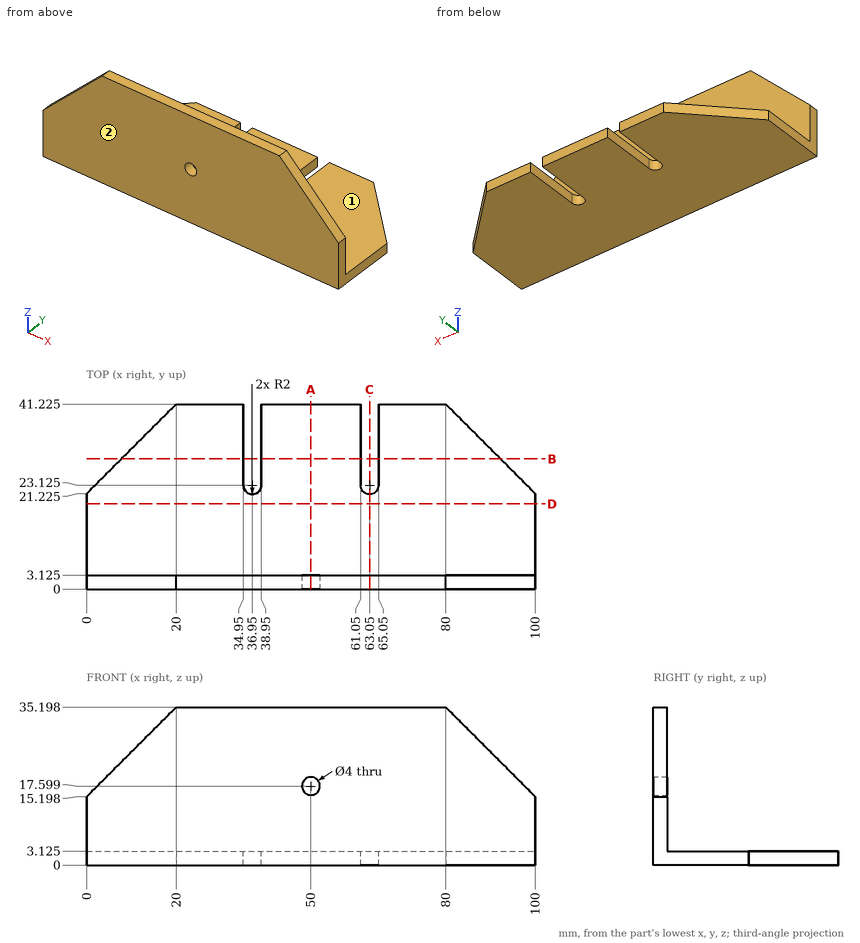
Geometry check sheet. Reference: drawing and pictorial views, mm from the part's lowest x, y, z. A direction names the side the tool comes from. Coordinates: 2 decimals unless noted, no trailing zeros. Write each loop counter-clockwise with the first axis right and the second up, starting at its lowest first coordinate (ties: lowest second). Pieces come first, ordered by that corner, then holes.
Item 1: Cross-section at C-C on x = 63.05. Record the boundary of the cut face in (y, z) (3 decimals), then the cut area to 3 significant figures.
Numbers:
outline: (0, 0) - (21.125, 0) - (21.125, 3.125) - (3.125, 3.125) - (3.125, 35.198) - (0, 35.198) - close
area: 166 mm2
Item 2: Scan line: probe 1 along Z at (x, y) = (49, 16) (3 decimals). Record every from-to range of solid material in increasing order.
Numbers:
probe 1: z = 0 to 3.125
Item 3: Cross-section at A-A on x = 50. Record the boundary of the cut face in (y, z) (3 decimals).
Numbers:
outline: (0, 0) - (41.225, 0) - (41.225, 3.125) - (3.125, 3.125) - (3.125, 15.599) - (0, 15.599) - close; (0, 19.599) - (3.125, 19.599) - (3.125, 35.198) - (0, 35.198) - close
Item 4: Cross-section at B-B on y = 29. Record the boundary of the cut face in (x, z) (3 decimals).
Numbers:
outline: (7.775, 0) - (34.95, 0) - (34.95, 3.125) - (7.775, 3.125) - close; (38.95, 0) - (61.05, 0) - (61.05, 3.125) - (38.95, 3.125) - close; (65.05, 0) - (92.225, 0) - (92.225, 3.125) - (65.05, 3.125) - close
Item 5: Cross-section at D-D on y = 19. Record the boundary of the cut face in (x, z) (3 decimals), then the cut area to 4 significant figures.
Numbers:
outline: (0, 0) - (100, 0) - (100, 3.125) - (0, 3.125) - close
area: 312.5 mm2
Item 6: Depth check by flat-ended pin: pin 1 Ø3 at (x, y) = (46, 36.5) entering from +Z (3 decimals); pin 2 Ø1.6 at (y, z) = (30.5, 1.5) entering from +X (3 decimals); pin 3 Ø3.5 at (y, z) = (30.5, 1) entering from -X (3 decimals). Enter the tip coordinate at first touch or a pass-through.
Numbers:
pin 1: stops at z = 3.125
pin 2: stops at x = 91.525
pin 3: stops at x = 7.525
Item 7: Access from +Z, -Z, +X, -X, +Y, -Y to the whole of each face (thin tool, end or side, straight path). Record for the marked faces 1 and 2.
Numbers:
face 1: +Z, +X, -X, +Y
face 2: +Z, -Z, +X, -X, -Y
